CAD build for the part. Positions are in the model's coordinates, mm. A direction names the side the tool comes from. Coordinates: 2 decimals unless noted, no trailing zeros. Loops run counter-clockwise (first coordinate to the right, second up) from the corner with the lowest first, then second, coordinate; pieces in that order, holes last.
1) Saw through at C-C, the plane y = 5. Write the cut outline in (x, z).
2) Saw through at A-A, the plane z = -5. Write the cut outline in (x, y).
3) Saw through at B-B, the plane x = 3.5. Write the cut outline in (y, z), and give its area (3 significant figures).
4) Which spindle directions (+Z, -Z, +X, -X, +Y, -Y) get a long thin tool onto all of the face, cutting with end or side? Do faces 1 (the flat face through (0, 5, -12)), 2 (the cylindrical face through (-0.285, 0.301, -12.521)), 3 (the flat face through (1, 0, -3)), 4 (the cylindrical face through (4.699, 9.715, -5.056)). Say none if no direction does.
5) Saw through at D-D, the plane y = 8.25. Write the cut outline in (x, z), and give its area (3 significant figures).
6) Wall check: line 1 along Y through (x, z) = (-1.5, -5); line 2 along X through (y, z) = (6.25, -11.75); line 3 along Z through (x, y) = (8.5, 8.5). Give the ranges that are in metal, low to high.
7) Pin check, flat tips, straight feed: pin 1 Ø4 at (x, z) = (6.5, -0.5) entering from -Y; pin 2 Ø2.5 at (x, y) = (11, 6) entering from -Z; pin 3 Ø4 at (y, z) = (6.5, -5.5) entering from +X; pin 4 Ø0.9 at (y, z) = (7, -12.5) entering from +X. Stop position of each tip, or through.
Autodesk Inventor part; units mm, degrees
ref_plane "YZ Plane" through (0, 0, 0) normal (1, 0, 0) x (0, 1, 0)
ref_plane "XZ Plane" through (0, 0, 0) normal (0, 1, 0) x (-1, 0, 0)
ref_plane "XY Plane" through (0, 0, 0) normal (0, 0, 1) x (1, 0, 0)
sketch "Sketch2" plane through (0, 0, 0) normal (0, 1, 0) x (-1, 0, 0)
  line L0 (0, 0) -> (0, -15)
  line L1 (0, 0) -> (-15, 0)
  line L2 (0, -15) -> (5, -15)
  line L3 (5, -15) -> (5, 5)
  line L4 (5, 5) -> (-15, 5)
  line L5 (-15, 5) -> (-15, 0)
  dimension "d0" = 15
  dimension "d1" = 15
  dimension "d3" = 5
  dimension "d4" = 20
  dimension "d5" = 90
  dimension "d6" = 20
extrude "Extrusion1" add sketch "Sketch2" along normal blind 10
sketch "Sketch3" plane through (0, 0, 0) normal (1, 0, 0) x (0, 0, -1)
  line L0 (15, 0) -> (15, 10) construction
  line L1 (15, 5) -> (-5, 5) construction
  circle A0 centre (5, 5) radius 2.5
  line L2 (0, 0) -> (15, 0)
  line L3 (0, 10) -> (15, 10)
  line L4 (0, 0) -> (10, 0)
  line L5 (10, 0) -> (10, 10)
  line L6 (10, 10) -> (0, 10)
  line L7 (0, 10) -> (0, 0)
  dimension "d9" = 5
  dimension "d10" = 10
  dimension "d17" = 10
extrude "Extrusion2" cut sketch "Sketch3" against normal blind 5 contours A0
extrude "Extrusion3" add sketch "Sketch3" along normal blind 5
fillet "Fillet2" radius 1 24 edges at (5, 5, -10) (5, 10, -5) (5, 0, -5) (10, 10, 0) (5, 5, 0) (10, 0, 0) (15, 5, 0) (15, 10, 2.5) (15, 0, 2.5) (15, 5, 5) (2.5, 10, -10) (0, 10, -12.5) (0, 5, -10) (0, 0, -12.5) (0, 5, -15) (-5, 5, -15) (-2.5, 10, -15) (-2.5, 0, -15) (5, 10, 5) (-5, 10, -5) (2.5, 0, -10) (5, 0, 5) (-5, 0, -5) (-5, 5, 5)
properties part number "support" material "Plastic, Opaque Black"
Data:
1. outline: (-5, -14) arc R1 ccw to (-4, -15) - (-1, -15) arc R1 ccw to (0, -14) - (0, -11) arc R1 cw to (1, -10) - (4, -10) arc R1 ccw to (5, -9) - (5, -7.5) - (-5, -7.5) - close; (-5, -2.5) - (5, -2.5) - (5, -1) arc R1 cw to (6, 0) - (14, 0) arc R1 ccw to (15, 1) - (15, 4) arc R1 ccw to (14, 5) - (-4, 5) arc R1 ccw to (-5, 4) - close
2. outline: (-5, 1) arc R1 ccw to (-4, 0) - (4, 0) arc R1 ccw to (5, 1) - (5, 2.5) - (-5, 2.5) - close; (-5, 7.5) - (5, 7.5) - (5, 9) arc R1 ccw to (4, 10) - (-4, 10) arc R1 ccw to (-5, 9) - close
3. outline: (0, -9) arc R1 ccw to (1, -10) - (9, -10) arc R1 ccw to (10, -9) - (10, 4) arc R1 ccw to (9, 5) - (1, 5) arc R1 ccw to (0, 4) - close; hole circle Ø5 at (5, -5)
3. area: 130 mm2
4. face 1: -Z, +X, +Y, -Y
4. face 2: -Z, +X, -Y
4. face 3: +Z, -Z, +X, -X, -Y
4. face 4: -Z, +X, +Y
5. outline: (-5, -14) arc R1 ccw to (-4, -15) - (-1, -15) arc R1 ccw to (0, -14) - (0, -11) arc R1 cw to (1, -10) - (4, -10) arc R1 ccw to (5, -9) - (5, -1) arc R1 cw to (6, 0) - (14, 0) arc R1 ccw to (15, 1) - (15, 4) arc R1 ccw to (14, 5) - (-4, 5) arc R1 ccw to (-5, 4) - close
5. area: 224 mm2
6. line 1: y = 0 to 2.5, 7.5 to 10
6. line 2: x = -5 to 0
6. line 3: z = 0 to 5
7. pin 1: stops at y = 0
7. pin 2: stops at z = 0
7. pin 3: stops at x = 5
7. pin 4: stops at x = 0
